Could you check a few things on this model? Use its own coordinates, in mm. Face numbers are marked on the shaded views. A direction names the side the tool comes from. Give positions to 0.01 mm unless a question says otherwise; leave off trailing zeros. Loops run counter-clockwise (first coordinate to the right, second up) from the corner with the lowest first, then second, coordinate; pieces in that order, holes last.
1. I need wall thicknesses on line 1 along Z through (x, y) = (28.5, -13.5); line 2 along X through (y, z) = (26.5, 0.5); line 3 along X through (y, z) = (35.5, 8.75). Which ranges of each line are inside material? Lowest first, please.
2. For the marked faces 1 and 2, which set-ups out of +Z, -Z, +X, -X, +Y, -Y let a thin tool reach every point of the face, with its end or its side?
3. Imagine slicing it at B-B (y = -10.5). List the corners of the cut face in (x, z) for me.
4. Imagine slicing it at A-A (x = 0). List the corners of the cut face in (y, z) for me, plus the area to 3 significant figures.
5. Thinking about a two-plate mould opening in X: for the marked faces 3, 4 and 5, which applies, +X half, -X half, draft (parallel to the pull), parting line (faces both ways), or undercut?
6. Imagine slicing it at D-D (x = 30.5). List the corners of the cut face in (y, z) for me, plus the area to 3 significant figures.
7. Imagine slicing it at C-C (z = 12.25). List the corners of the cut face in (x, y) for me, plus the area to 3 significant figures.
8. For P1, Ø2, axis at x = 29.5, z = 4.5, coming from the +Y side; P2, Ø1, axis at x = 14, z = 4, coming from the -Y side; P3, Ø5, axis at x = 41, z = 2.5, coming from the +Y side, each with a flat end and sliding along its axis, tell me the tip position at first contact or that it passes through.
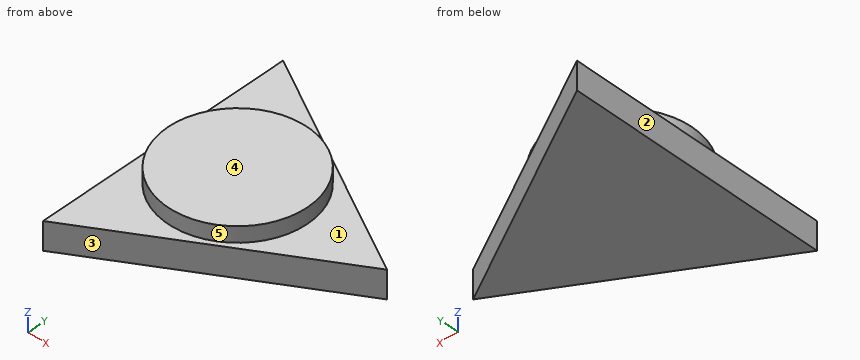
```python
from build123d import *

# Parameters (mm, degrees)
F1_DEPTH = 10.23828
F2_R     = 25.715841
F3_DEPTH = 5.69966


with BuildPart() as f1:
    # F0 (on Top) → F1 (new body)
    with BuildSketch(Plane.XY):
        Polygon((-27.506582, 47.642798), (-27.506582, -47.642798), (55.013165, 0), align=None)
    extrude(amount=F1_DEPTH)

    # F2 (on face) → F3 (join)
    with BuildSketch(Plane.XY.offset(10.23828)):
        Circle(F2_R)
    extrude(amount=F3_DEPTH)


solid = f1.part
```
Derived:
1. line 1: z = 0 to 10.24
1. line 2: x = -27.51 to 9.11
1. line 3: x = -27.51 to -6.47
2. face 1: +Z
2. face 2: +Z, -Z, -X, +Y, -Y
3. outline: (-27.51, 0) - (36.83, 0) - (36.83, 10.24) - (23.47, 10.24) - (23.47, 15.94) - (-23.47, 15.94) - (-23.47, 10.24) - (-27.51, 10.24) - close
4. outline: (-31.76, 0) - (31.76, 0) - (31.76, 10.24) - (25.72, 10.24) - (25.72, 15.94) - (-25.72, 15.94) - (-25.72, 10.24) - (-31.76, 10.24) - close
4. area: 944 mm2
5. face 3: +X half
5. face 4: draft
5. face 5: parting line
6. outline: (-14.15, 0) - (14.15, 0) - (14.15, 10.24) - (-14.15, 10.24) - close
6. area: 290 mm2
7. outline: circle Ø51.43 at (0, 0)
7. area: 2,080 mm2
8. P1: stops at y = 15.31
8. P2: stops at y = -23.97
8. P3: stops at y = 9.53
